The model under review builds one solid part; all positions refer to its coordinate system, in mm. Face numbers are marked on the shaded views. A direction names the side the tool comes from. Give positions to 0.01 mm unless a question says otherwise; leave off trailing zeros. Order: outer loops, then holes, each group sorted by start corner. A loop starts at its lowest first (then second) coordinate and runs counter-clockwise, first axis right, second up. Notation, with made-up numbers: (86.5, -14) -> (109.5, -14) arc R21 ccw to (109.5, -3) -> close; hole circle Ø5 at (77, 76). An arc over 180 degrees is marked (long way). Answer as a JSON object with one key per item and string values. Group by question number.
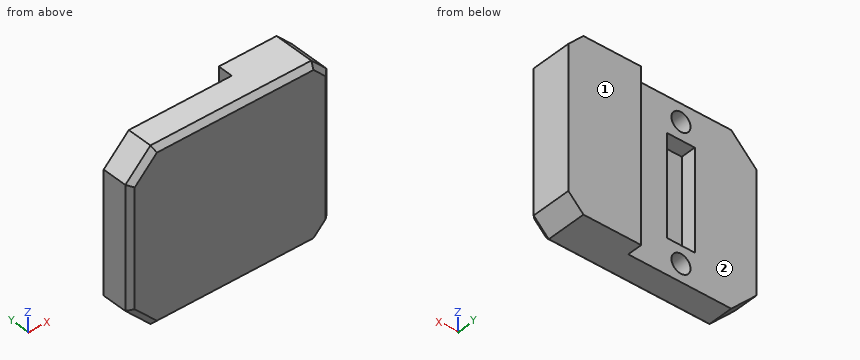
from build123d import *

# Parameters (mm, degrees)
CYLINDER016013_R                  = 1.9
CYLINDER016013_DEPTH              = 10
CYLINDER016014_R                  = 1.9
CYLINDER016014_DEPTH              = 10
BOX018_W                          = 5.5
BOX018_H                          = 3
BOX018_DEPTH                      = 20
BOX016_W                          = 25.5
BOX016_H                          = 3
BOX016_DEPTH                      = 34
BOX017_W                          = 40
BOX017_H                          = 9
BOX017_DEPTH                      = 34
CHAMFER016016008004017002011_SIZE = 5
CHAMFER016016008004017002012_SIZE = 3
CHAMFER016016008004017002013_SIZE = 1


with BuildPart() as cylinder029:
    # Cylinder016013 → Cylinder016013 (new body)
    with BuildSketch(Plane(origin=(-15, 0, 3.5), x_dir=(1, 0, 0), z_dir=(0, 1, 0))):
        Circle(CYLINDER016013_R)
    extrude(amount=CYLINDER016013_DEPTH)


with BuildPart() as fusion018002:
    # Cylinder016014 → Cylinder016014 (new body)
    with BuildSketch(Plane(origin=(-15, 0, 30.5), x_dir=(1, 0, 0), z_dir=(0, 1, 0))):
        Circle(CYLINDER016014_R)
    extrude(amount=CYLINDER016014_DEPTH)

    # Fusion018002: union Cylinder029
    add(cylinder029.part)


with BuildPart() as fusion018002_1:
    # Fusion018002 placement: moved
    add(fusion018002.part.moved(Location((0, -8, 0))))


with BuildPart() as cube018:
    # Box018 → Box018 (new body)
    with BuildSketch(Plane(origin=(-17.75, -7, 7), x_dir=(1, 0, 0), z_dir=(0, 0, 1))):
        with Locations((2.75, 1.5)):
            Rectangle(BOX018_W, BOX018_H)
    extrude(amount=BOX018_DEPTH)


with BuildPart() as cube016:
    # Box016 → Box016 (new body)
    with BuildSketch(Plane(origin=(-30, -4, 0), x_dir=(1, 0, 0), z_dir=(0, 0, 1))):
        with Locations((12.75, 1.5)):
            Rectangle(BOX016_W, BOX016_H)
    extrude(amount=BOX016_DEPTH)


with BuildPart() as obj1:
    # Box017 → Box017 (new body)
    with BuildSketch(Plane(origin=(-30, -10, 0), x_dir=(1, 0, 0), z_dir=(0, 0, 1))):
        with Locations((20, 4.5)):
            Rectangle(BOX017_W, BOX017_H)
    extrude(amount=BOX017_DEPTH)

    # Cut010011008003: cut Cube016
    add(cube016.part, mode=Mode.SUBTRACT)

    # Cut010011008009003016015: cut Cube018
    add(cube018.part, mode=Mode.SUBTRACT)

    # Cut010011008009003016016: cut Fusion018002
    add(fusion018002_1.part, mode=Mode.SUBTRACT)

    # Chamfer016016008004017002011
    chamfer016016008004017002011_edges = [obj1.edges().sort_by_distance(p)[0] for p in [
        (-30, -7, 34),
        (-30, -7, 0),
    ]]
    chamfer(chamfer016016008004017002011_edges, length=CHAMFER016016008004017002011_SIZE)

    # Chamfer016016008004017002012
    chamfer016016008004017002012_edges = [obj1.edges().sort_by_distance(p)[0] for p in [
        (10, -5.5, 0),
        (10, -5.5, 34),
    ]]
    chamfer(chamfer016016008004017002012_edges, length=CHAMFER016016008004017002012_SIZE)

    # Chamfer016016008004017002013
    chamfer016016008004017002013_edges = [obj1.edges().sort_by_distance(p)[0] for p in [
        (-9, -10, 0),
        (-27.5, -10, 2.5),
        (-30, -10, 17),
        (-27.5, -10, 31.5),
        (-9, -10, 34),
        (8.5, -10, 32.5),
        (10, -10, 17),
        (8.5, -10, 1.5),
    ]]
    chamfer(chamfer016016008004017002013_edges, length=CHAMFER016016008004017002013_SIZE)


solid = obj1.part
1. Take a section at D-D on y = -9.5. Give the boundary of the cut face in (x, z), plus the area to 3 significant figures.
2. For probe 1 along Z at (x, y) = (-15, -7.1); probe 2 along Z at (x, y) = (-15, -5.45); probe 3 along Z at (x, y) = (-26, -4.5), list the stretches that pass through material, from the lowest coordinate up. Write a range as [from, to].
3. For pin 1 (6 mm diameter, centred on x = -15, z = 30.5, fed in from +Y); pin 2 (1.1 mm diameter, centred on x = -15.5, z = 31, fed in from +Y); pin 3 (1.6 mm diameter, centred on x = -14, z = 18.5, fed in from +Y), all flat-tipped, find the tip position at first contact; note any pin that passes through.
4. Take a section at A-A on z = 20.5. Give the boundary of the cut face in (x, y).
5. Take a section at C-C on y = -7.5. Give the boundary of the cut face in (x, z), plus the area to 3 significant figures.
6. Machinability: for the marked faces 1 and 2, which of the approach directions +Z, -Z, +X, -X, +Y, -Y give a long, thin tool a straight path to every point of the face, cutting with its end or side? Answer none if there is none.
7. Take a section at B-B on x = -15. Give the boundary of the cut face in (y, z).
Checks:
{
 "1": {"outline": "(-29.5, 5.21) -> (-24.79, 0.5) -> (6.79, 0.5) -> (9.5, 3.21) -> (9.5, 30.79) -> (6.79, 33.5) -> (-24.79, 33.5) -> (-29.5, 28.79) -> close", "area": "1,260 mm2"},
 "2": {"probe 1": "z = [0, 1.6], [5.4, 28.6], [32.4, 34]", "probe 2": "z = [0, 1.6], [5.4, 7], [27, 28.6], [32.4, 34]", "probe 3": "z = [1, 33]"},
 "3": {"pin 1": "stops at y = -4", "pin 2": "stops at y = -8", "pin 3": "stops at y = -7"},
 "4": {"outline": "(-30, -9) -> (-29, -10) -> (9, -10) -> (10, -9) -> (10, -1) -> (-4.5, -1) -> (-4.5, -4) -> (-12.25, -4) -> (-12.25, -7) -> (-17.75, -7) -> (-17.75, -4) -> (-30, -4) -> close"},
 "5": {"outline": "(-30, 5) -> (-25, 0) -> (7, 0) -> (10, 3) -> (10, 31) -> (7, 34) -> (-25, 34) -> (-30, 29) -> close; hole circle Ø3.8 at (-15, 3.5); hole circle Ø3.8 at (-15, 30.5)", "area": "1,300 mm2"},
 "6": {"face 1": "+Z, -Z, +X, -X, +Y", "face 2": "+Z, -Z, -X, +Y"},
 "7": {"outline": "(-10, 1) -> (-9, 0) -> (-4, 0) -> (-4, 1.6) -> (-8, 1.6) -> (-8, 5.4) -> (-4, 5.4) -> (-4, 7) -> (-7, 7) -> (-7, 27) -> (-4, 27) -> (-4, 28.6) -> (-8, 28.6) -> (-8, 32.4) -> (-4, 32.4) -> (-4, 34) -> (-9, 34) -> (-10, 33) -> close"}
}
